from build123d import *

# Parameters (mm, degrees)
SKETCH009_W     = 54.5
SKETCH009_H     = 15
PAD003_DEPTH    = 14
SKETCH011_R     = 5
PAD005_DEPTH    = 10
SKETCH012_R     = 3.4
POCKET004_DEPTH = 30


with BuildPart() as part:
    # Sketch009 → Pad003 (new body)
    with BuildSketch(Plane.XY):
        with Locations((-27.25, 7.5)):
            Rectangle(SKETCH009_W, SKETCH009_H)
    extrude(amount=PAD003_DEPTH)

    # Sketch011 (on Face3 of Pad003) → Pad005 (join)
    with BuildSketch(Plane(origin=(0, 15, 0), x_dir=(-1, 0, 0), z_dir=(0, 1, 0))):
        with Locations((27.25, 7)):
            Circle(SKETCH011_R)
    extrude(amount=PAD005_DEPTH)

    # Sketch012 (on Face8 of Pad005) → Pocket004 (cut)
    with BuildSketch(Plane(origin=(0, 25, 0), x_dir=(-1, 0, 0), z_dir=(0, 1, 0))):
        with Locations((27.25, 7)):
            Circle(SKETCH012_R)
    extrude(amount=-POCKET004_DEPTH, mode=Mode.SUBTRACT)


solid = part.part
Geometry check sheet. Reference: the model listing, model coordinates, mm. Give positions to 0.01 mm unless a question says otherwise; leave off trailing zeros. Write each loop counter-clockwise with the first axis right and the second up, starting at its lowest first coordinate (ties: lowest second). Pieces come first, ordered by that corner, then holes.
1) Cross-section at A-A (x = -27.25). Record the boundary of the cut face in (y, z), plus the area to 3 significant figures.
Values follow:
outline: (0, 0) - (15, 0) - (15, 2) - (25, 2) - (25, 3.6) - (0, 3.6) - close; (0, 10.4) - (25, 10.4) - (25, 12) - (15, 12) - (15, 14) - (0, 14) - close
area: 140 mm2
2) Go/stop test with flat-tipped pins: pin 1 Ø8 at (x, z) = (-16.5, 6.5) entering from +Y; pin 2 Ø4 at (x, z) = (-27.25, 7) entering from -Y. Record where each tip stops, or that it passes through.
Values follow:
pin 1: stops at y = 15
pin 2: passes through
3) Cross-section at B-B (z = 7). Record the boundary of the cut face in (x, y), plus the area to 4 significant figures.
Values follow:
outline: (-54.5, 0) - (-30.65, 0) - (-30.65, 25) - (-32.25, 25) - (-32.25, 15) - (-54.5, 15) - close; (-23.85, 0) - (0, 0) - (0, 15) - (-22.25, 15) - (-22.25, 25) - (-23.85, 25) - close
area: 747.5 mm2
4) Cross-section at D-D (y = 19). Record the boundary of the cut face in (x, z).
Values follow:
outline: circle Ø10 at (-27.25, 7); hole circle Ø6.8 at (-27.25, 7)
5) Thickness scan on line 1 (Z direction, x = -27.25, y = 9.5); line 2 (Z direction, x = -27.25, y = 16.75); line 3 (Y direction, x = -1.5, z = 5.75). Record the ranges inside material, lowest first.
Values follow:
line 1: z = 0 to 3.6, 10.4 to 14
line 2: z = 2 to 3.6, 10.4 to 12
line 3: y = 0 to 15
6) Release check for a two-part mould opening along X. For faces 1 (the face through (-54.5, 7, 7)), 2 (the face through (-30.39, 12.68, 5.7)), 3 (the face through (-28, 0, 2)), 4 (the face through (-22.255, 19.93, 7.22)) record: released by +X, released by -X, zero draft, split by the parting line, or undercut.
Values follow:
face 1: released by -X
face 2: undercut
face 3: zero draft
face 4: split by the parting line
7) Cross-section at C-C (y = 12.75). Record the boundary of the cut face in (x, z).
Values follow:
outline: (-54.5, 0) - (0, 0) - (0, 14) - (-54.5, 14) - close; hole circle Ø6.8 at (-27.25, 7)
